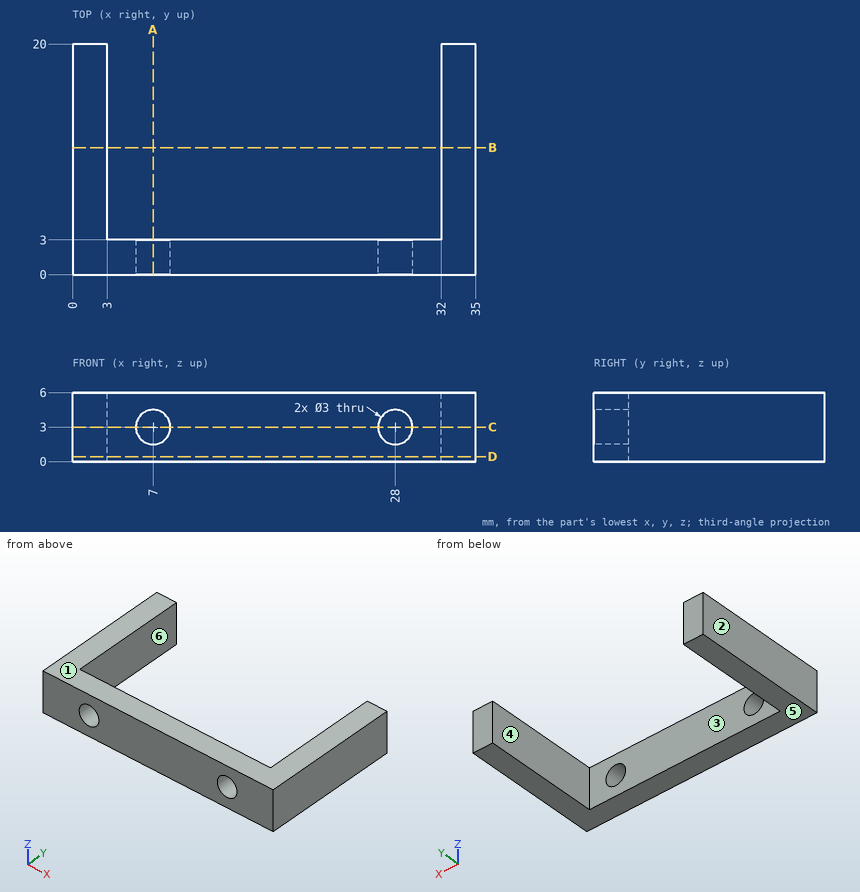
Verification items for this drawing (mm, ordinates from the low corner). A direction names the side the tool comes from. Coordinates: 2 decimals unless noted, no trailing zeros. Order: outer loops, then holes, each group sorted by start corner. A loop starts at its lowest first (then second) coordinate and runs counter-clockwise, first axis right, second up. Notation, with made-up numbers: M 73,30 L 104,30 A16 ccw 104,52 Z; hole C -1.5,-12 d4. An arc over 180 degrees is marked long. One line per item, written item: value. Start each with the question number.
Item 1: Mould release check, pull along X, two halves, no side actions. Record for the marked faces 1, 2, 3 and 4: pulls with the +X half, pulls with the -X half, needs draft (parallel to the pull), parting line crosses it, or undercut.
Item 2: Sectioned sample at A-A on x = 7. Record the cut outline in (y, z), then the cut area to 3 significant figures.
Item 3: Access from +Z, -Z, +X, -X, +Y, -Y to the whole of each face (thin tool, end or side, straight path). Record for the marked faces 5 and 6.
Item 4: Thickness scan on probe 1 along X at (y, z) = (11.75, 0.5); probe 2 along Z at (x, y) = (28, 1.95); probe 3 along Y at (x, z) = (5, 3.7). Record the ranges inside material, lowest first.
Item 5: Sectioned sample at B-B on y = 11. Record the cut outline in (x, z).
Item 6: Sectioned sample at C-C on z = 3. Record the cut outline in (x, y), then the cut area to 3 significant figures.
Item 7: Sectioned sample at D-D on z = 0.45. Record the cut outline in (x, y), then the cut area to 3 significant figures.
Item 8: Depth check by flat-ended pin: P1, Ø6, axis at x = 8, y = 5, coming from the +Z side; P2, Ø3.5, axis at x = 28, z = 3, coming from the +Y side. Enter the tip coordinate at first touch or a pass-through.
Calculated:
1. face 1: needs draft
1. face 2: pulls with the -X half
1. face 3: undercut
1. face 4: undercut
2. outline: M 0,0 L 3,0 L 3,1.5 L 0,1.5 Z; M 0,4.5 L 3,4.5 L 3,6 L 0,6 Z
2. area: 9.00 mm^2
3. face 5: -Z, +X, -X, +Y, -Y
3. face 6: +Z, -Z, +Y
4. probe 1: 0 to 3, 32 to 35
4. probe 2: 0 to 1.5, 4.5 to 6
4. probe 3: 0 to 3
5. outline: M 0,0 L 3,0 L 3,6 L 0,6 Z; M 32,0 L 35,0 L 35,6 L 32,6 Z
6. outline: M 0,0 L 5.5,0 L 5.5,3 L 3,3 L 3,20 L 0,20 Z; M 8.5,0 L 26.5,0 L 26.5,3 L 8.5,3 Z; M 29.5,0 L 35,0 L 35,20 L 32,20 L 32,3 L 29.5,3 Z
6. area: 189 mm^2
7. outline: M 0,0 L 35,0 L 35,20 L 32,20 L 32,3 L 3,3 L 3,20 L 0,20 Z
7. area: 207 mm^2
8. P1: z = 6
8. P2: y = 3
